Drawing for the job (mm, zero at the part's lowest x, y, z). A direction names the side the tool comes from. Round coordinates to 2 decimals unless told otherwise and drop trailing zeros. Loops run counter-clockwise (first coordinate to the right, second up) from the corner with the lowest first, then second, coordinate; pieces in that order, holes last. Notation, with made-up numbers: (-11, 19) -> (26, 19) arc R16 ccw to (26, 40) -> close; hole circle Ø4 at (78, 45). An arc over 180 degrees is marked (long way). Put each result on its own line as item: value. Start each with the question number.
Item 1: Cut at C-C, the plane x = 26. List the corners of the cut face in (y, z), plus the area to 3 significant figures.
Item 2: Drill centre lines: probe 1 along X at (y, z) = (4.5, 26); probe 2 along Z at (x, y) = (26, 1.5); probe 3 along X at (y, z) = (1.05, 12). Where is each one in solid material? Low to high. Write a range as [from, to].
Item 3: Pull direction X, two halves, no side cores. Call the marked faces 5, 6, 7 and 8: +X half, -X half, draft (parallel to the pull), parting line (faces both ways), or undercut.
Item 4: Cut at B-B, the plane y = 4. List the corners of the cut face in (x, z).
Item 5: Cut at D-D, the plane z = 26. List the corners of the cut face in (x, y), plus the area to 3 significant figures.
Item 6: Cut at A-A, the plane x = 18.5. List the corners of the cut face in (y, z).
Item 7: Flat gauge pins, fed straight in: pin 1 Ø1.5 at (y, z) = (4, 15.5) entering from -X; pin 2 Ø1.5 at (x, y) = (8.5, 4.5) entering from +Z; pin 3 Ø3.5 at (x, y) = (27, 2) entering from -Z; pin 4 Ø1.5 at (y, z) = (1.5, 39) entering from -X. Where does each tip first touch, or does it go through?
Item 8: Tool access for the marked faces 1, 2, 3 and 4: list every direction of +Z, -Z, +X, -X, +Y, -Y with a clear straight run to the whole face (end or side of a thin tool).
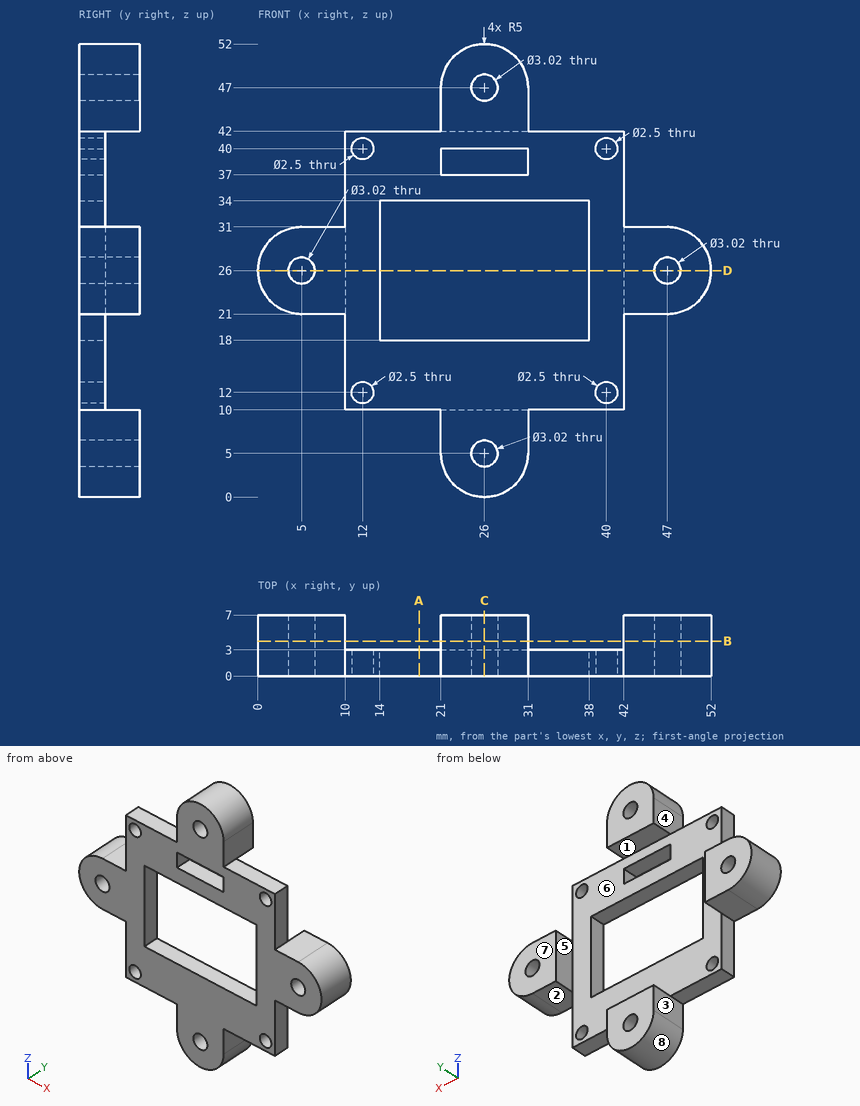
Reply:
1. outline: (0, 0) -> (7, 0) -> (7, 3.49) -> (0, 3.49) -> close; (0, 6.51) -> (7, 6.51) -> (7, 10) -> (3, 10) -> (3, 18) -> (0, 18) -> close; (0, 34) -> (3, 34) -> (3, 37) -> (0, 37) -> close; (0, 40) -> (3, 40) -> (3, 42) -> (7, 42) -> (7, 45.49) -> (0, 45.49) -> close; (0, 48.51) -> (7, 48.51) -> (7, 52) -> (0, 52) -> close
1. area: 137 mm^2
2. probe 1: x = [0, 3.49], [6.51, 10], [42, 45.49], [48.51, 52]
2. probe 2: z = [0, 3.49], [6.51, 18], [34, 37], [40, 45.49], [48.51, 52]
2. probe 3: x = [10, 10.75], [13.25, 38.75], [41.25, 42]
3. face 5: undercut
3. face 6: undercut
3. face 7: draft
3. face 8: parting line
4. outline: (5, 21) -> (10, 21) -> (10, 31) -> (5, 31) arc R5 ccw to start; (21, 5) arc R5 ccw to (31, 5) -> (31, 10) -> (21, 10) -> close; (21, 42) -> (31, 42) -> (31, 47) arc R5 ccw to (21, 47) -> close; (42, 21) -> (47, 21) arc R5 ccw to (47, 31) -> (42, 31) -> close; hole circle Ø3.02 at (5, 26); hole circle Ø3.02 at (26, 5); hole circle Ø3.02 at (26, 47); hole circle Ø3.02 at (47, 26)
5. outline: (0, 0) -> (3.49, 0) -> (3.49, 7) -> (0, 7) -> close; (6.51, 0) -> (14, 0) -> (14, 3) -> (10, 3) -> (10, 7) -> (6.51, 7) -> close; (38, 0) -> (45.49, 0) -> (45.49, 7) -> (42, 7) -> (42, 3) -> (38, 3) -> close; (48.51, 0) -> (52, 0) -> (52, 7) -> (48.51, 7) -> close
5. area: 122 mm^2
6. outline: (0, 10) -> (3, 10) -> (3, 18) -> (0, 18) -> close; (0, 34) -> (3, 34) -> (3, 42) -> (0, 42) -> close
7. pin 1: passes through
7. pin 2: stops at z = 31
7. pin 3: stops at z = 0
7. pin 4: stops at x = 10
8. face 1: +X, -X, +Y
8. face 2: -Z, +X, +Y, -Y
8. face 3: -Z, -X, +Y, -Y
8. face 4: +Z, -X, +Y, -Y
